The model under review builds one solid part; all positions refer to its coordinate system, in mm. Round coordinates to 2 decimals unless told otherwise and drop trailing zeros. Write each loop counter-clockwise with the first axis right and the second up, starting at its lowest first coordinate (ties: lowest second). Pieces come first, ordered by that corner, then holes. Notation, with made-up numbers: (5.25, 70) - (30.25, 70) arc R35 cw to (30.25, 103) - close; hole circle Ø2 at (16, -2). An arc over 180 degrees is marked (long way). Return JSON: item names as keys, results as strings.
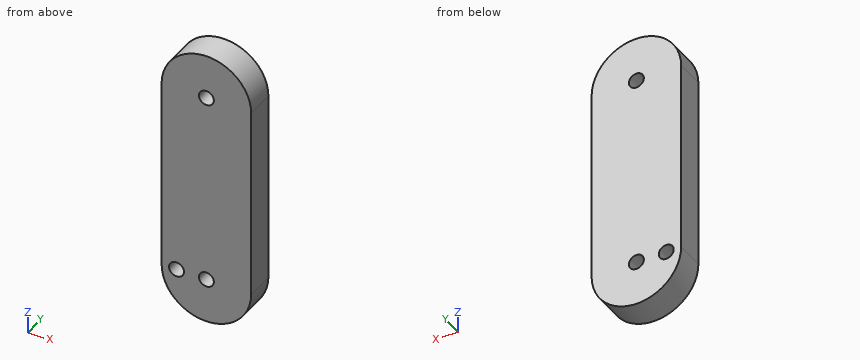
from build123d import *

# Parameters (mm, degrees)
EXTRUDE_1_DEPTH          = 10
CUT_EXTRUDE_1_DEPTH      = 87.02325267
CUT_EXTRUDE_1_DEPTH_BACK = 87.02325267
SKETCH_2_R               = 2.5
SKETCH_4_R               = 2.5
CUT_EXTRUDE_3_DEPTH      = 10


with BuildPart() as part:
    # 草图1 → 凸台-拉伸1 (new body)
    with BuildSketch(Plane(origin=(0, 0, 0), x_dir=(1, 0, 0), z_dir=(0, 1, 0))):
        with BuildLine():
            Line((0, 0), (0, 65))
            ThreePointArc((0, 65), (15, 80), (30, 65))
            Line((30, 65), (30, 0))
            ThreePointArc((30, 0), (15, -15), (0, 0))
        make_face()
    extrude(amount=EXTRUDE_1_DEPTH)

    # 草图2 → 切除-拉伸1 (cut, two sides: drawn at the far end of the back side and taken through both)
    with BuildSketch(Plane(origin=(0, 10, 0), x_dir=(1, 0, 0), z_dir=(0, 1, 0)).offset(-CUT_EXTRUDE_1_DEPTH_BACK)):
        with Locations(Location((15, 65, 0), (0, 0, 270))):
            Circle(SKETCH_2_R)
        with Locations(Location((15, 0, 0), (0, 0, 90))):
            Circle(SKETCH_2_R)
    extrude(amount=CUT_EXTRUDE_1_DEPTH + CUT_EXTRUDE_1_DEPTH_BACK, mode=Mode.SUBTRACT)

    # 草图4 → 切除-拉伸3 (cut)
    with BuildSketch(Plane(origin=(0, 10, 0), x_dir=(1, 0, 0), z_dir=(0, 1, 0))):
        with Locations(Location((5, 65, 0), (0, 0, 270))):
            Circle(SKETCH_4_R)
    extrude(amount=-CUT_EXTRUDE_3_DEPTH, mode=Mode.SUBTRACT)


solid = part.part
(1) Add section A-A (x = 15). Write out the cut boundary in (y, z).
Filled in:
{"outline": "(0, -80) - (10, -80) - (10, -67.5) - (0, -67.5) - close; (0, -62.5) - (10, -62.5) - (10, -2.5) - (0, -2.5) - close; (0, 2.5) - (10, 2.5) - (10, 15) - (0, 15) - close"}
(2) Wall thickness on line 1 (X direction, y = 2.75, z = -65); line 2 (Z direction, x = 14.5, y = 2.75); line 3 (Z direction, x = 6.75, y = 3): over which ranges is each line inside the solid? List them lowest first.
Filled in:
{"line 1": "x = 0 to 2.5, 7.5 to 12.5, 17.5 to 30", "line 2": "z = -79.99 to -67.45, -62.55 to -2.45, 2.45 to 14.99", "line 3": "z = -77.53 to -66.79, -63.21 to 12.53"}
(3) Clearance check with flat-ended pins moving along their axes: pin 1 Ø4 at (x, y) = (7.5, 7) entering from -Z; pin 2 Ø4 at (x, z) = (15, 0) entering from +Y; pin 3 Ø1.5 at (x, y) = (24.5, 4.5) entering from +Z; pin 4 Ø1 at (x, y) = (19, 3) entering from -Z. State where each tip first meets the part, or that it passes through.
Filled in:
{"pin 1": "stops at z = -78.96", "pin 2": "passes through", "pin 3": "stops at z = 12.18", "pin 4": "stops at z = -79.59"}
(4) Add section D-D (x = 27). Write out the cut boundary in (y, z), plus the area to 3 significant figures.
Filled in:
{"outline": "(0, -74) - (10, -74) - (10, 9) - (0, 9) - close", "area": "830 mm2"}
(5) Add section B-B (y = 3.75). Write out the cut boundary in (x, z).
Filled in:
{"outline": "(0, -65) arc R15 ccw to (30, -65) - (30, 0) arc R15 ccw to (0, 0) - close; hole circle Ø5 at (5, -65); hole circle Ø5 at (15, -65); hole circle Ø5 at (15, 0)"}
(6) Add section C-C (x = 5). Write out the cut boundary in (y, z).
Filled in:
{"outline": "(0, -76.18) - (10, -76.18) - (10, -67.5) - (0, -67.5) - close; (0, -62.5) - (10, -62.5) - (10, 11.18) - (0, 11.18) - close"}
